Part model, mm, in its own coordinate system. A direction names the side the tool comes from. Give positions to 0.01 mm unless a question says otherwise; leave off trailing zeros. Write each loop counter-clockwise with the first axis right and the second up, starting at its lowest first coordinate (ties: lowest second). Pieces come first, ordered by that corner, then holes. Notation, with made-up numbers: (26.5, 72) - (75.5, 72) arc R14 cw to (75.5, 89) - close; hole circle Ø11 at (24.25, -25). An arc over 180 degrees is marked (long way). Answer as a JSON object with one key per item and string values. Group by question number.
```python
from build123d import *

# Parameters (mm, degrees)
SKETCH1_W           = 25
SKETCH1_H           = 25
BOSS_EXTRUDE1_DEPTH = 4
SKETCH2_W           = 20
SKETCH2_H           = 20
CUT_EXTRUDE1_DEPTH  = 3
SKETCH3_R           = 1.25
BOSS_EXTRUDE2_DEPTH = 2
FILLET1_R           = 1
SKETCH4_R           = 1
BOSS_EXTRUDE3_DEPTH = 2


with BuildPart() as part:
    # Sketch1 → Boss-Extrude1 (new body)
    with BuildSketch(Plane(origin=(0, 0, 0), x_dir=(1, 0, 0), z_dir=(0, 1, 0))):
        Rectangle(SKETCH1_W, SKETCH1_H)
    extrude(amount=BOSS_EXTRUDE1_DEPTH)

    # Sketch2 → Cut-Extrude1 (cut)
    with BuildSketch(Plane(origin=(0, 4, 0), x_dir=(1, 0, 0), z_dir=(0, 1, 0))):
        Rectangle(SKETCH2_W, SKETCH2_H)
    extrude(amount=-CUT_EXTRUDE1_DEPTH, mode=Mode.SUBTRACT)

    # Sketch3 → Boss-Extrude2 (add)
    with BuildSketch(Plane(origin=(0, 1, 0), x_dir=(1, 0, 0), z_dir=(0, 1, 0))):
        Circle(SKETCH3_R)
    extrude(amount=BOSS_EXTRUDE2_DEPTH)

    # Fillet1
    fillet1_edges = [part.edges().sort_by_distance(p)[0] for p in [
        (-1.25, 3, 0),
    ]]
    fillet(fillet1_edges, radius=FILLET1_R)

    # Sketch4 → Boss-Extrude3 (add)
    with BuildSketch(Plane(origin=(0, 4, 0), x_dir=(1, 0, 0), z_dir=(0, 1, 0))):
        with Locations((-11, 11)):
            Circle(SKETCH4_R)
        with Locations((11, 11)):
            Circle(SKETCH4_R)
        with Locations((11, -11)):
            Circle(SKETCH4_R)
        with Locations((-11, -11)):
            Circle(SKETCH4_R)
    extrude(amount=BOSS_EXTRUDE3_DEPTH)


solid = part.part
```
1) Mould opens along X. For faces 3 (the flat face through (2, 1, 0)), 4 (the flat face through (12.5, 2, 0)), 5 (the flat face through (-12.5, 2, 0)), 6 (the flat face through (0, 2, 12.5)) say: pulls with the +X half, pulls with the -X half, needs draft (parallel to the pull), parting line crosses it, or undercut.
2) Probe line 1 (Z direction, x = 3, y = 3.75); line 2 (Y direction, x = 10.25, z = -2.5). List the from-to ranges inside material, lowest first.
3) Drop flat-ended pins along their axis: P1, Ø12.5, axis at x = 6, z = 4.5, coming from the +Y side; P2, Ø0.6, axis at x = 0, z = 0, coming from the +Y side. Give the stop position or say it passes through.
4) Which spindle directions (+Z, -Z, +X, -X, +Y, -Y) get a long thin tool onto all of the face, cutting with end or side? Do faces 1 (the cylindrical face through (10.2, 5, -10.4)), 2 (the flat face through (11, 6, -11)). Say none if no direction does.
5) Band-saw the part on B-B (x = -8.5). List the corners of the cut face in (y, z).
6) Band-saw the part on A-A (y = 3.3). List the corners of the cut face in (x, z).
7) Band-saw the part on C-C (y = 5). List the corners of the cut face in (x, z).
8) Band-saw the part on D-D (z = 2.75). List the corners of the cut face in (x, y), plus the area to 3 significant figures.
Verdict:
{
 "1": {"face 3": "undercut", "face 4": "pulls with the +X half", "face 5": "pulls with the -X half", "face 6": "needs draft"},
 "2": {"line 1": "-12.5 to -10, 10 to 12.5", "line 2": "0 to 4"},
 "3": {"P1": "y = 4", "P2": "y = 3"},
 "4": {"face 1": "+Y", "face 2": "+Z, -Z, +X, -X, +Y"},
 "5": {"outline": "(0, -12.5) - (4, -12.5) - (4, -10) - (1, -10) - (1, 10) - (4, 10) - (4, 12.5) - (0, 12.5) - close"},
 "6": {"outline": "(-12.5, -12.5) - (12.5, -12.5) - (12.5, 12.5) - (-12.5, 12.5) - close; hole (-10, -10) - (10, -10) - (10, 10) - (-10, 10) - close"},
 "7": {"outline": "circle Ø2 at (-11, -11); circle Ø2 at (-11, 11); circle Ø2 at (11, -11); circle Ø2 at (11, 11)"},
 "8": {"outline": "(-12.5, 0) - (12.5, 0) - (12.5, 4) - (10, 4) - (10, 1) - (-10, 1) - (-10, 4) - (-12.5, 4) - close", "area": "40.0 mm2"}
}
